Verification items for the finished model (mm, model axes). Face numbers are marked on the shaded views. Give positions to 0.01 mm unless a question says otherwise; leave off trailing zeros. Write each loop counter-clockwise with the first axis right and the second up, starting at its lowest first coordinate (ties: lowest second). Pieces come first, ordered by that corner, then holes. Notation, with made-up numbers: (69.5, 67.25) -> (77.5, 67.25) arc R15 ccw to (77.5, 84.25) -> close; hole circle Ø7 at (80.25, 32.5). An arc over 180 degrees is marked (long way). Use one line per item in the form item = value. Start each with the question number.
(1) Section check A-A, the plane x = 0. Record the cut outline in (y, z) (3 decimals).
(2) Section check C-C, the plane z = 1.65. Record the cut outline in (x, y) (3 decimals), plus the area to 3 significant figures.
(3) Release check for a two-part mould opening along Y. For the marked faces 1, 2 and 3 record: pulls with the +Y half, pulls with the -Y half, needs draft (parallel to the pull), parting line crosses it, or undercut.
(4) Scan lines: L1, parallel to Y at x = 0, z = 0.45 (3 decimals); L2, parallel to Y at x = 0, z = 1.7 (3 decimals); L3, parallel to X at y = 0, z = 0.25 (3 decimals). Record each from-to range of solid material in increasing order.
(5) Section check B-B, the plane y = 0. Record the cut outline in (x, z) (3 decimals).
(6) Depth check by flat-ended pin: pin 1 Ø1 at (x, y) = (0, 0) entering from -Z (3 decimals). Enter the tip coordinate at first touch or a pass-through.
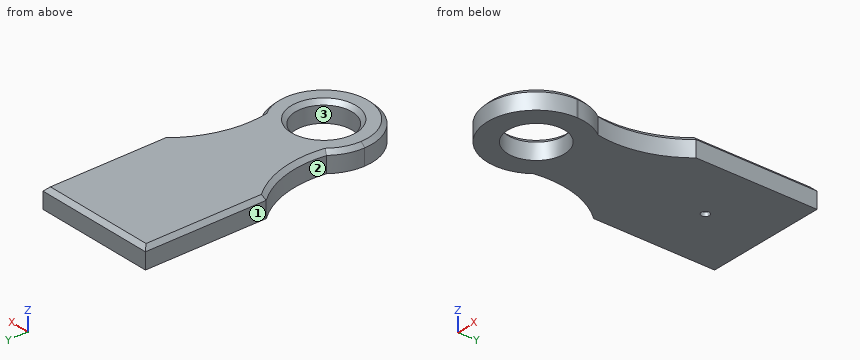
from build123d import *

# Parameters (mm, degrees)
F0_W       = 19.05
F0_H       = 19.05
F0_R       = 4.445
F1_DEPTH   = 3.175
F2_C1_SIZE = 0.635
F2_C2_SIZE = 0.635
F2_C3_SIZE = 0.635
F2_C4_SIZE = 0.635
F2_C5_SIZE = 0.635
F2_C6_SIZE = 0.635
F2_C7_SIZE = 0.6349
F3_R       = 0.635
F4_DEPTH   = 0.635


# Not quite as in the source:
# - a fillet or chamfer is up to 0.001 mm smaller than in the source, because OpenCascade refuses the exact size


with BuildPart() as f1:
    # F0 (on Top) → F1 (new body)
    with BuildSketch(Plane.XY):
        Rectangle(F0_W, F0_H)
        with BuildLine():
            Line((9.525, -9.525), (-9.525, -9.525))
            ThreePointArc((-9.525, -9.525), (-6.3836187271, -15.3786997104), (-6.0310725347, -22.012687032))
            ThreePointArc((-6.0310725347, -22.012687032), (0.0350329382, -19.0500805324), (6.0736411029, -22.0683390224))
            ThreePointArc((6.0736411029, -22.0683390224), (6.3936440411, -15.409890989), (9.525, -9.525))
        make_face()
        with BuildLine():
            ThreePointArc((6.0736411029, -22.0683390224), (0.0350329382, -19.0500805324), (-6.0310725347, -22.012687032))
            ThreePointArc((-6.0310725347, -22.012687032), (-6.6363180101, -24.4058987838), (-7.62, -26.67))
            ThreePointArc((-7.62, -26.67), (0, -34.29), (7.62, -26.67))
            ThreePointArc((7.62, -26.67), (7.619882327, -26.6276523681), (7.6195293118, -26.5853060441))
            ThreePointArc((7.6195293118, -26.5853060441), (6.6686101992, -24.3877327559), (6.0736411029, -22.0683390224))
        make_face()
        with Locations((0, -26.67)):
            Circle(F0_R, mode=Mode.SUBTRACT)
        with BuildLine():
            ThreePointArc((-7.62, -26.67), (-6.6363180101, -24.4058987838), (-6.0310725347, -22.012687032))
            ThreePointArc((-6.0310725347, -22.012687032), (-7.2118365454, -24.2095501137), (-7.62, -26.67))
        make_face()
        with BuildLine():
            ThreePointArc((7.6195293118, -26.5853060441), (7.2094713239, -24.202628275), (6.0736411029, -22.0683390224))
            ThreePointArc((6.0736411029, -22.0683390224), (6.6686101992, -24.3877327559), (7.6195293118, -26.5853060441))
        make_face()
    extrude(amount=F1_DEPTH)

    # F2: chamfer of 0.635 on 7 edges, made by hand

    # F2_c1
    f2_c1_edges = [f1.edges().sort_by_distance(p)[0] for p in [
        (0, 9.525, 3.175),
    ]]
    chamfer(f2_c1_edges, length=F2_C1_SIZE)

    # F2_c2
    f2_c2_edges = [f1.edges().sort_by_distance(p)[0] for p in [
        (-9.525, -0.3175, 3.175),
    ]]
    chamfer(f2_c2_edges, length=F2_C2_SIZE)

    # F2_c3
    f2_c3_edges = [f1.edges().sort_by_distance(p)[0] for p in [
        (-6.2554888364, -15.867774564, 3.175),
    ]]
    chamfer(f2_c3_edges, length=F2_C3_SIZE)

    # F2_c4
    f2_c4_edges = [f1.edges().sort_by_distance(p)[0] for p in [
        (6.3936440411, -15.409890989, 3.175),
    ]]
    chamfer(f2_c4_edges, length=F2_C4_SIZE)

    # F2_c5
    f2_c5_edges = [f1.edges().sort_by_distance(p)[0] for p in [
        (9.525, 0.1573240758, 3.175),
    ]]
    chamfer(f2_c5_edges, length=F2_C5_SIZE)

    # F2_c6
    f2_c6_edges = [f1.edges().sort_by_distance(p)[0] for p in [
        (-4.445, -26.67, 3.175),
    ]]
    chamfer(f2_c6_edges, length=F2_C6_SIZE)

    # F2_c7 (size 0.635 in the source; OpenCascade refuses exactly that, so slightly less here)
    f2_c7_edges = [f1.edges().sort_by_distance(p)[0] for p in [
        (-0.0350329382, -34.2899194676, 3.175),
    ]]
    chamfer(f2_c7_edges, length=F2_C7_SIZE)

    # F3 (on face) → F4 (cut)
    with BuildSketch(Plane(origin=(0, 0, 0), x_dir=(1, 0, 0), z_dir=(0, 0, -1))):
        Circle(F3_R)
    extrude(amount=-F4_DEPTH, mode=Mode.SUBTRACT)


solid = f1.part
Completed:
q1.outline = (-34.29, 0) -> (-31.115, 0) -> (-31.115, 2.54) -> (-31.75, 3.175) -> (-33.655, 3.175) -> (-34.29, 2.54) -> close; (-22.225, 0) -> (-0.635, 0) -> (-0.635, 0.635) -> (0.635, 0.635) -> (0.635, 0) -> (9.525, 0) -> (9.525, 2.54) -> (8.89, 3.175) -> (-21.59, 3.175) -> (-22.225, 2.54) -> close
q2.outline = (-9.525, -9.525) arc R15.24 cw to (-6.031, -22.013) arc R7.62 ccw (long way) to (7.62, -26.67) arc R7.62 ccw to (7.62, -26.585) arc R7.62 ccw to (6.074, -22.068) arc R15.24 cw to (9.525, -9.525) -> (9.525, 9.525) -> (-9.525, 9.525) -> close; hole circle Ø8.89 at (0, -26.67)
q2.area = 628 mm²
q3.face_1 = needs draft
q3.face_2 = undercut
q3.face_3 = undercut
q4.L1 = -34.29 to -31.115, -22.225 to -0.635, 0.635 to 9.525
q4.L2 = -34.29 to -31.115, -22.225 to 9.525
q4.L3 = -9.525 to -0.635, 0.635 to 9.525
q5.outline = (-9.525, 0) -> (-0.635, 0) -> (-0.635, 0.635) -> (0.635, 0.635) -> (0.635, 0) -> (9.525, 0) -> (9.525, 2.54) -> (8.89, 3.175) -> (-8.89, 3.175) -> (-9.525, 2.54) -> close
q6.pin_1 = 0.635
